from build123d import *

# Parameters (mm, degrees)
SKETCH1_W           = 43
SKETCH1_H           = 150
BOSS_EXTRUDE1_DEPTH = 4
SKETCH2_W           = 10.57
SKETCH2_H           = 21.1
SKETCH2_W_2         = 10.75
CUT_EXTRUDE1_DEPTH  = 79.123299982
CUT_EXTRUDE2_DEPTH  = 2.5
SKETCH4_R           = 1.75
CUT_EXTRUDE3_DEPTH  = 79.123299982


with BuildPart() as part:
    # Sketch1 → Boss-Extrude1 (new body)
    with BuildSketch(Plane(origin=(0, 0, 0), x_dir=(1, 0, 0), z_dir=(0, 1, 0))):
        Rectangle(SKETCH1_W, SKETCH1_H)
    extrude(amount=BOSS_EXTRUDE1_DEPTH)

    # Sketch2 → Cut-Extrude1 (cut, through all)
    with BuildSketch(Plane(origin=(0, 4, 0), x_dir=(1, 0, 0), z_dir=(0, 1, 0))):
        with Locations((5.285, 64.45)):
            Rectangle(SKETCH2_W, SKETCH2_H)
        with Locations((-5.375, 64.45)):
            Rectangle(SKETCH2_W_2, SKETCH2_H)
    extrude(amount=-CUT_EXTRUDE1_DEPTH, mode=Mode.SUBTRACT)

    # Sketch3 → Cut-Extrude2 (cut)
    with BuildSketch(Plane(origin=(0, 4, 0), x_dir=(1, 0, 0), z_dir=(0, 1, 0))):
        Polygon((-15.25, 31.654101615), (-18.25, 29.922050808), (-18.25, 26.457949192), (-15.25, 24.725898385), (-12.25, 26.457949192), (-12.25, 29.922050808), align=None)
        Polygon((12.25, 29.922050808), (15.25, 31.654101615), (18.25, 29.922050808), (18.25, 26.457949192), (15.25, 24.725898385), (12.25, 26.457949192), align=None)
        Polygon((12.25, -0.577949192), (12.25, -4.042050808), (15.25, -5.774101615), (18.25, -4.042050808), (18.25, -0.577949192), (15.25, 1.154101615), align=None)
        Polygon((-12.25, -4.042050808), (-15.25, -5.774101615), (-18.25, -4.042050808), (-18.25, -0.577949192), (-15.25, 1.154101615), (-12.25, -0.577949192), align=None)
    extrude(amount=-CUT_EXTRUDE2_DEPTH, mode=Mode.SUBTRACT)

    # Sketch4 → Cut-Extrude3 (cut, through all)
    with BuildSketch(Plane(origin=(0, 4, 0), x_dir=(1, 0, 0), z_dir=(0, 1, 0))):
        with Locations(Location((-15.25, 28.19, 0), (0, 0, 270))):
            Circle(SKETCH4_R)
        with Locations(Location((15.25, 28.19, 0), (0, 0, 90))):
            Circle(SKETCH4_R)
        with Locations(Location((15.25, -2.31, 0), (0, 0, 270))):
            Circle(SKETCH4_R)
        with Locations(Location((-15.25, -2.31, 0), (0, 0, 90))):
            Circle(SKETCH4_R)
    extrude(amount=-CUT_EXTRUDE3_DEPTH, mode=Mode.SUBTRACT)


solid = part.part
Geometry check sheet. Reference: the model listing, model coordinates, mm. A direction names the side the tool comes from. Give positions to 0.01 mm unless a question says otherwise; leave off trailing zeros. Order: outer loops, then holes, each group sorted by start corner. A loop starts at its lowest first (then second) coordinate and runs counter-clockwise, first axis right, second up. Notation, with made-up numbers: M 62.5,69.25 L 75.5,69.25 A22 ccw 75.5,78.25 Z; hole C -22.5,-5 d7. An arc over 180 degrees is marked long. Use a Markdown table: item, result.
Item 1: Depth check by flat-ended pin: P1, Ø3, axis at x = -15.25, z = 2.31, coming from the -Y side; P2, Ø4.5, axis at x = 15.25, z = -28.19, coming from the -Y side; P3, Ø2, axis at x = 2.5, y = 2, coming from the -Z side. Enter the tip coordinate at first touch or a pass-through.
Answers follow:
| item | result |
|---|---|
| P1 | passes through |
| P2 | stops at y = 0 |
| P3 | stops at z = -53.9 |
Item 2: Material ranges on line 1 along X through (y, z) = (0.3, 2.31); line 2 along X through (y, z) = (1.95, 2.5); line 3 along Z through (x, y) = (15.5, 2.1), recorded low to high.
Answers follow:
| item | result |
|---|---|
| line 1 | x = -21.5 to -17, -13.5 to 13.5, 17 to 21.5 |
| line 2 | x = -21.5 to -18.25, -12.25 to 12.25, 18.25 to 21.5 |
| line 3 | z = -75 to -31.51, -24.87 to -1.01, 5.63 to 75 |
Item 3: Section check B-B (y = 0.8). Record the cut outline in (x, z), and give its area (3 significant figures).
Answers follow:
| item | result |
|---|---|
| outline | M -21.5,-75 L -10.75,-75 L -10.75,-53.9 L 10.57,-53.9 L 10.57,-75 L 21.5,-75 L 21.5,75 L -21.5,75 Z; hole C -15.25,-28.19 d3.5; hole C -15.25,2.31 d3.5; hole C 15.25,-28.19 d3.5; hole C 15.25,2.31 d3.5 |
| area | 5,960 mm2 |
Item 4: Section check C-C (x = -6). Record the cut outline in (y, z).
Answers follow:
| item | result |
|---|---|
| outline | M 0,-53.9 L 4,-53.9 L 4,75 L 0,75 Z |
Item 5: Tool access check on faces 3 (the flat face through (13.729, 2.768, -30.776)), 4 (the cylindrical face through (-16.985, 0.76, 2.538)), 5 (the flat face through (-10.75, 2, -64)). Record the directions out of +Z, -Z, +X, -X, +Y, -Y that give a thin tool (end or side, any length) a straight path to the whole face; none if there is none.
Answers follow:
| item | result |
|---|---|
| face 3 | +Y |
| face 4 | +Y, -Y |
| face 5 | -Z, +Y, -Y |
Item 6: Draft check along X on faces 1 (the flat face through (16.771, 2.768, -0.276)), 2 (the flat face through (0, 4, -1)). Enter one of: +X half, -X half, draft (parallel to the pull), parting line (faces both ways), or undercut.
Answers follow:
| item | result |
|---|---|
| face 1 | undercut |
| face 2 | draft |
Item 7: Section check A-A (z = -28.19). Record the cut outline in (x, y), and give its area (4 significant figures).
Answers follow:
| item | result |
|---|---|
| outline | M -21.5,0 L -17,0 L -17,1.5 L -18.25,1.5 L -18.25,4 L -21.5,4 Z; M -13.5,0 L 13.5,0 L 13.5,1.5 L 12.25,1.5 L 12.25,4 L -12.25,4 L -12.25,1.5 L -13.5,1.5 Z; M 17,0 L 21.5,0 L 21.5,4 L 18.25,4 L 18.25,1.5 L 17,1.5 Z |
| area | 131.5 mm2 |
